Design review of the part shown in the three views and the two pictorial views. Dimensions are in mm from the part's minimum x, y and z. A direction names the side the tool comes from. Coordinates: 2 decimals unless noted, no trailing zeros. Loops run counter-clockwise (first coordinate to the right, second up) from the corner with the lowest first, then second, coordinate; pieces in that order, holes last. Notation, with made-up numbers: (54, -38.5) -> (75, -38.5) arc R10 cw to (75, -33.5) -> close; hole circle Ø7 at (50, 17). An arc over 180 degrees is marked (long way). Answer in a Markdown table with one row per item.
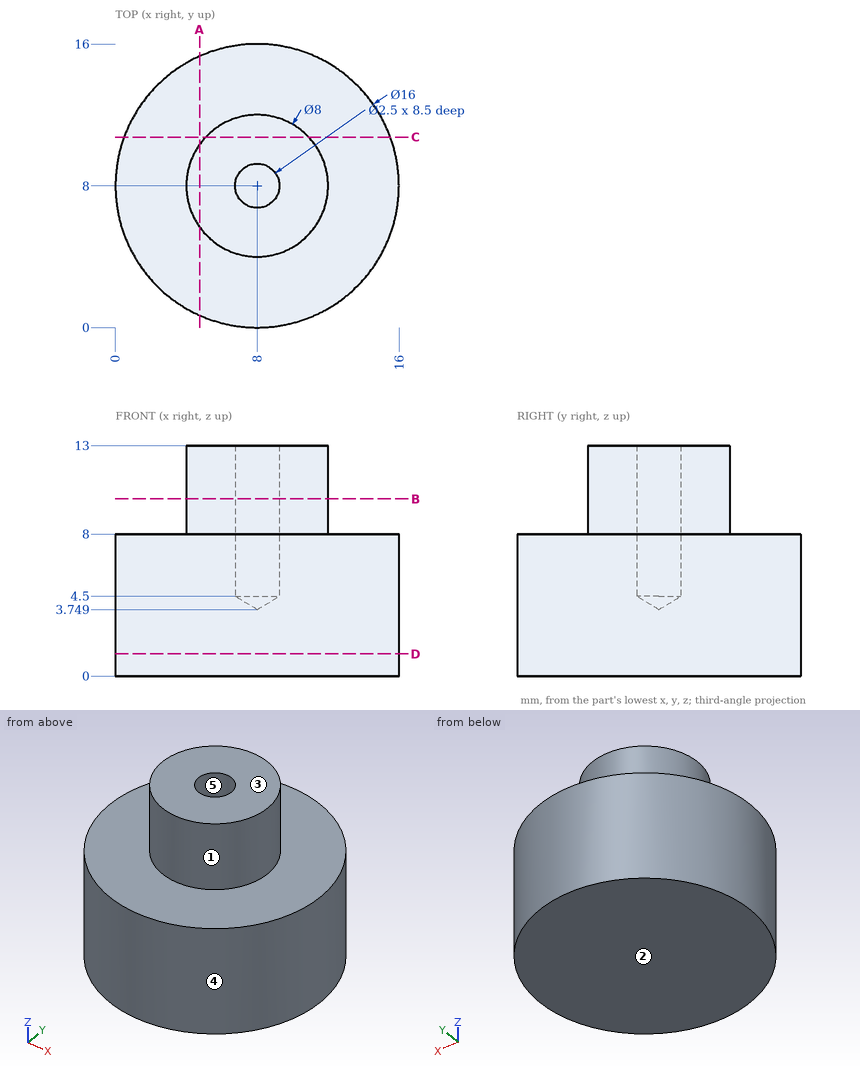
Item 1: The part is to be moulded in two halves that separate along Y. For the marked faces 3, 4 and 5, say which applies: +Y half, -Y half, draft (parallel to the pull), parting line (faces both ways), or undercut.
Worked answers:
| item | result |
|---|---|
| face 3 | draft |
| face 4 | parting line |
| face 5 | undercut |
Item 2: Take a section at B-B, the plane z = 10. State the section outline as (x, y) points, and give its area (3 significant figures).
Worked answers:
| item | result |
|---|---|
| outline | circle Ø8 at (8, 8); hole circle Ø2.5 at (8, 8) |
| area | 45.4 mm² |
Item 3: Take a section at C-C, the plane y = 10.75. State the section outline as (x, z) points, and give its area (3 significant figures).
Worked answers:
| item | result |
|---|---|
| outline | (0.49, 0) -> (15.51, 0) -> (15.51, 8) -> (10.9, 8) -> (10.9, 13) -> (5.1, 13) -> (5.1, 8) -> (0.49, 8) -> close |
| area | 149 mm² |
Item 4: For L1, parallel to Y at x = 8, z = 11.25; L2, parallel to Y at x = 8, z = 7.75; L3, parallel to Z at x = 14.75, y = 6.75, list the stretches that pass through material, from the lowest coordinate up.
Worked answers:
| item | result |
|---|---|
| L1 | 4 to 6.75, 9.25 to 12 |
| L2 | 0 to 6.75, 9.25 to 16 |
| L3 | 0 to 8 |
Item 5: Take a section at D-D, the plane z = 1.25. State the section outline as (x, y) points.
Worked answers:
| item | result |
|---|---|
| outline | circle Ø16 at (8, 8) |
Item 6: Take a section at A-A, the plane x = 4.75. State the section outline as (y, z) points, and give its area (3 significant figures).
Worked answers:
| item | result |
|---|---|
| outline | (0.69, 0) -> (15.31, 0) -> (15.31, 8) -> (10.33, 8) -> (10.33, 13) -> (5.67, 13) -> (5.67, 8) -> (0.69, 8) -> close |
| area | 140 mm² |
Item 7: Insertion check: pin 1 (4 mm diameter, centred on y = 11, z = 9.5, fed in from +X); pin 2 (1 mm diameter, centred on y = 6, z = 5, fed in from -X); pin 3 (5 mm diameter, centred on x = 3.5, z = 3.5, fed in from -Y). Each pin has a flat end and moves straight along its axis. Give the tip position at first contact, or say it passes through.
Worked answers:
| item | result |
|---|---|
| pin 1 | x = 15.82 |
| pin 2 | x = 0.14 |
| pin 3 | y = 0.25 |
Item 8: For the marked faces 1 and 2, list the 3-axis set-ups (+Z, -Z, +X, -X, +Y, -Y) from which the entire face can be reached by the end or side of a thin tool; tool diameter is ignored.
Worked answers:
| item | result |
|---|---|
| face 1 | +Z |
| face 2 | -Z, +X, -X, +Y, -Y |
